Source: CAD feature listing. Evaluate the final solid. Frame: model axes, mm. A direction names the side the tool comes from. Round coordinates to 2 decimals unless told otherwise and drop trailing zeros. Loops run counter-clockwise (first coordinate to the right, second up) from the corner with the lowest first, then second, coordinate; pieces in that order, holes last. Notation, with made-up numbers: (3, 84.25) - (23, 84.25) arc R30 cw to (23, 115.25) - close; hole circle Ø6 at (0.5, 57). An arc over 180 degrees is marked (long way). One line per question, with ' | ' between items. Start each with the question number.
1. Ray query, line 1 (Z direction, x = 20, y = -3); line 2 (Y direction, x = 29.5, z = -52.5); line 3 (X direction, y = 217.5, z = -65.5). Return the intervals inside material, ascending.
2. Cut plane A-A (z = -65.5). Return loops of the section in (x, y).
3. Cut plane B-B (y = 154.5). Return loops of the section in (x, z).
4. Access query for faces 1 (the flat face through (78, 245, -75)), 2 (the flat face through (75, 121, -75)). Directions: +Z, -Z, +X, -X, +Y, -Y. A direction counts if a zero-diameter tool reaches every point of the face in a straight line with its end or side. Return the directions, or none.
5. Pin query (flat end, axial travel): pin 1 (1 mm diameter, centred on y = 95.5, z = -79.5, fed in from -X); pin 2 (25 mm diameter, centred on x = 50.5, z = -78.5, fed in from +Y); pin 3 (2 mm diameter, centred on x = 60, z = -79.53, fed in from +Y). Return the tip coordinate at first contact, or that it passes through.
```python
from build123d import *

# Parameters (mm, degrees)
F0_W     = 80
F0_H     = 50
F0_R     = 1.65
F1_DEPTH = 5
F2_W     = 245
F2_H     = 50
F3_DEPTH = 5


with BuildPart() as f1:
    # F0 (on Front) → F1 (new body)
    with BuildSketch(Plane.XZ):
        with Locations((40, -75)):
            Rectangle(F0_W, F0_H)
        with Locations((20, -79.52825)):
            Circle(F0_R, mode=Mode.SUBTRACT)
        with Locations((60, -79.52825)):
            Circle(F0_R, mode=Mode.SUBTRACT)
    extrude(amount=F1_DEPTH)

    # F2 (on face) → F3 (join)
    with BuildSketch(Plane.YZ.offset(80)):
        with Locations((122.5, -75)):
            Rectangle(F2_W, F2_H)
    extrude(amount=-F3_DEPTH)


solid = f1.part
```
Answers follow:
1) line 1: z = -100 to -81.18, -77.88 to -50 | line 2: y = -5 to 0 | line 3: x = 75 to 80
2) outline: (0, -5) - (80, -5) - (80, 245) - (75, 245) - (75, 0) - (0, 0) - close
3) outline: (75, -100) - (80, -100) - (80, -50) - (75, -50) - close
4) face 1: +Z, -Z, +X, -X, +Y | face 2: +Z, -Z, -X, +Y
5) pin 1: stops at x = 75 | pin 2: stops at y = 0 | pin 3: passes through
